Model file for the job. Use its own axes, mm. A direction names the side the tool comes from. Coordinates: 2 decimals unless noted, no trailing zeros. Order: outer loops, then holes, each group sorted by start corner. A loop starts at its lowest first (then second) coordinate and runs counter-clockwise, first axis right, second up. Notation, with made-up numbers: M -14,53 L 39,53 A28 cw 39,77 Z; hole C 64.25,37 d3. An arc over 180 degrees is marked long. Return JSON: item names as keys, results as strings.
Autodesk Inventor part; units mm, degrees
ref_plane "YZ Plane" through (0, 0, 0) normal (1, 0, 0) x (0, 1, 0)
ref_plane "XZ Plane" through (0, 0, 0) normal (0, 1, 0) x (-1, 0, 0)
ref_plane "XY Plane" through (0, 0, 0) normal (0, 0, 1) x (1, 0, 0)
sketch "草圖1" plane through (0, 0, 0) normal (0, 0, 1) x (1, 0, 0)
  line L0 (-0.3223, -18.9936) -> (-5.7251, -18.9936)
  line L1 (-5.7251, -18.9936) -> (-5.7251, -20.1936)
  line L2 (-5.7251, -20.1936) -> (1.1777, -20.1936)
  line L3 (1.1777, -20.1936) -> (1.1777, -7.3911)
  line L4 (1.1777, -7.3911) -> (8.6477, -7.3911)
  line L5 (8.6477, -7.3911) -> (8.6477, -5.8911)
  line L6 (8.6477, -5.8911) -> (0.6777, -5.9936)
  line L7 (0.6777, -5.9936) -> (0.6777, -2.9936)
  line L8 (0.6777, -2.9936) -> (-0.3223, -2.9936)
  line L9 (-0.3223, -2.9936) -> (-0.3223, -18.9936)
  line L10 (0.6477, -6) -> (-0.2923, -6)
  line L11 (0.6477, 0) -> (0.6477, -6)
  line L12 (-0.2923, 0) -> (0.6477, 0)
  line L13 (-0.2923, 0) -> (-0.2923, -6)
  line L14 (4.1477, 0) -> (7.1477, 0)
  line L15 (4.1477, 0) -> (4.1477, -6)
  line L16 (7.1477, 0) -> (7.1477, -6)
  line L17 (7.1477, -6) -> (4.1477, -6)
  point P0 (0.1784, -6)
  point P1 (0.1777, -6)
  point P2 (8.6477, -6.6411)
  dimension "d0" = 1
  dimension "d3" = 0.94
  dimension "d4" = 0.03
  dimension "d5" = 3
  dimension "d6" = 1.5
  dimension "d7" = 1.2
  dimension "d8" = 16
  dimension "d9" = 1.5
  dimension "d10" = 1.5
extrude "擠出1" add sketch "草圖1" along normal blind 6 contours L9 L8 L13 L10 L11 L7 L6 L15 L17 L16 L5 L4 L3 L2 L1 L0 | L8 L11 L10 L13 | L6 L16 L17 L15
fillet "圓角1" radius 3 2 edges at (8.6477, -6.6411, 6) (8.6477, -6.6411, 0)
sketch "草圖3" plane through (0.6777, -5.9936, 6) normal (-0.0128564, 0.9999174, 0) x (0.9999174, 0.0128564, 0)
  ellipse E0 centre (5.0466, 3) end of major axis (5.0466, 1.5) minor radius 1.4999 construction
  ellipse E1 centre (4.9695, 3) end of major axis (4.9695, 4.5) minor radius 1.4999
  point P0 (-0.6006, 6)
extrude "擠出2" cut sketch "草圖3" against normal up to surface (1.4326 mm away)
equation "\"d4\" = -0.5 * d3 + 0.5 * d0"
properties part number "j1 enndstop blocker"
Item 1: Wall check: line 1 (Y direction, x = -5, z = 2.25); line 2 (X direction, y = -11, z = 5.75); line 3 (X direction, y = -4.5, z = 2.75). Give the ranges that are in metal, low to high.
Check result:
{"line 1": "y = -20.19 to -18.99", "line 2": "x = -0.32 to 1.18", "line 3": "x = -0.32 to 0.68"}
Item 2: Saw through at B-B (x = -3.5). Write the cut outline in (y, z), and give its area (3 significant figures).
Check result:
{"outline": "M -20.19,0 L -18.99,0 L -18.99,6 L -20.19,6 Z", "area": "7.20 mm2"}
Item 3: Saw through at A-A (z = 1). Write the cut outline in (x, y).
Check result:
{"outline": "M -5.73,-20.19 L 1.18,-20.19 L 1.18,-7.39 L 7.88,-7.39 L 7.88,-5.9 L 0.68,-5.99 L 0.68,-2.99 L -0.32,-2.99 L -0.32,-18.99 L -5.73,-18.99 Z"}
Item 4: Drop flat-ended pins along their axis: pin 1 Ø1.5 at (y, z) = (-5, 3) entering from +X; pin 2 Ø1.8 at (x, z) = (3, 2.5) entering from -Y; pin 3 Ø2 at (y, z) = (-15, 3) entering from +X. Give the stop position or say it passes through.
Check result:
{"pin 1": "stops at x = 0.68", "pin 2": "stops at y = -7.39", "pin 3": "stops at x = 1.18"}
Item 5: Saw through at C-C (y = -12.5). Write the cut outline in (x, z).
Check result:
{"outline": "M -0.32,0 L 1.18,0 L 1.18,6 L -0.32,6 Z"}
Item 6: 3-axis set-ups, long thin cutter, end or side, ignore diameter. For faces 1 (the flat face through (-0.322, -11, 3)), 2 (the flat face through (0, -2.994, 3)), 3 (the flat face through (4, -7.391, 3)): which of +Z, -Z, +X, -X, +Y, -Y reach the whole face in a straight line?
Check result:
{"face 1": "+Z, -Z, -X, +Y", "face 2": "+Z, -Z, +X, -X, +Y", "face 3": "+Z, -Z, +X, -Y"}
Item 7: Saw through at D-D (z = 5.5). Write the cut outline in (x, y).
Check result:
{"outline": "M -5.73,-20.19 L 1.18,-20.19 L 1.18,-7.39 L 7.31,-7.39 L 7.31,-5.91 L 0.68,-5.99 L 0.68,-2.99 L -0.32,-2.99 L -0.32,-18.99 L -5.73,-18.99 Z"}
